Read the model definition and answer for the solid it produces. Units are mm, in the model's axes. Face numbers are marked on the shaded views. Give positions to 0.01 mm unless a question says otherwise; leave off trailing zeros. Write each loop counter-clockwise with the first axis right and the second up, starting at its lowest first coordinate (ties: lowest second). Pieces come first, ordered by that corner, then holes. Notation, with made-up numbers: (67, -35.5) - (110, -35.5) arc R21 ccw to (110, -12.5) - close; hole circle Ø2 at (-12, 46). An arc over 180 degrees is marked (long way). Answer as CSV lines item,"result".
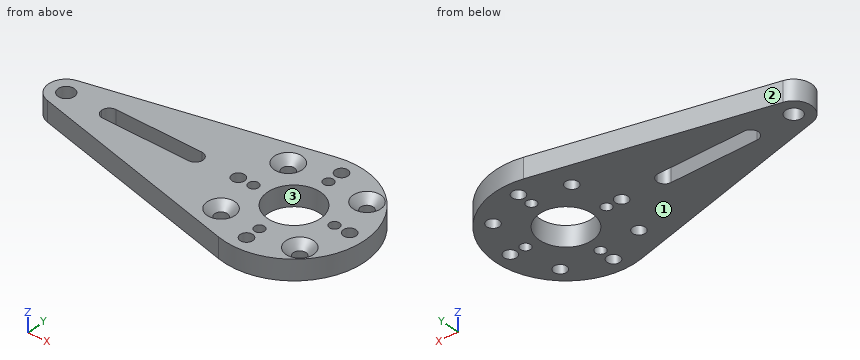
```python
from build123d import *

# Parameters (mm, degrees)
SKETCH1_R           = 1.6
SKETCH1_R_2         = 5.25
BOSS_EXTRUDE1_DEPTH = 4
CUT_EXTRUDE1_REACH  = 52.638
SKETCH2_R           = 1
CIRPATTERN1_COUNT   = 4
CUT_EXTRUDE2_REACH  = 52.638
SKETCH3_R           = 1.25
CIRPATTERN2_COUNT   = 8
CHAMFER1_SIZE       = 1.5
CUT_EXTRUDE3_REACH  = 52.638
SKETCH4_W           = 20
SKETCH4_H           = 3
FILLET1_R           = 1.5


with BuildPart() as part:
    # Sketch1 → Boss-Extrude1 (new body)
    with BuildSketch(Plane.XY):
        with BuildLine():
            Line((-45.816666667, 3.403388834), (-3.266666667, 13.613555336))
            ThreePointArc((-3.266666667, 13.613555336), (14, 0), (-3.266666667, -13.613555336))
            Line((-3.266666667, -13.613555336), (-45.816666667, -3.403388834))
            ThreePointArc((-45.816666667, -3.403388834), (-48.5, 0), (-45.816666667, 3.403388834))
        make_face()
        with Locations((-45, 0)):
            Circle(SKETCH1_R, mode=Mode.SUBTRACT)
        Circle(SKETCH1_R_2, mode=Mode.SUBTRACT)
    extrude(amount=BOSS_EXTRUDE1_DEPTH)

    # Sketch2 → Cut-Extrude1 (cut, up to next)
    with BuildSketch(Plane.XY.offset(4), mode=Mode.PRIVATE) as cut_extrude1_sk1:
        with Locations((0, 8)):
            Circle(SKETCH2_R)
    cut_extrude1_tool1 = extrude(cut_extrude1_sk1.sketch, amount=-CUT_EXTRUDE1_REACH, mode=Mode.PRIVATE) & part.part
    cut_extrude1 = cut_extrude1_tool1.solids().sort_by_distance((0, 8, 4))[0]
    add(cut_extrude1, mode=Mode.SUBTRACT)

    # CirPattern1: Cut-Extrude1 ×4 about axis
    cirpattern1_axis = Axis((0, 0, 0), (0, 0, 1))
    for i in range(1, CIRPATTERN1_COUNT):
        add(cut_extrude1.rotate(cirpattern1_axis, i * 360 / CIRPATTERN1_COUNT), mode=Mode.SUBTRACT)

    # Sketch3 → Cut-Extrude2 (cut, up to next)
    with BuildSketch(Plane.XY.offset(4), mode=Mode.PRIVATE) as cut_extrude2_sk1:
        with Locations((0, 11)):
            Circle(SKETCH3_R)
    cut_extrude2_tool1 = extrude(cut_extrude2_sk1.sketch, amount=-CUT_EXTRUDE2_REACH, mode=Mode.PRIVATE) & part.part
    cut_extrude2 = cut_extrude2_tool1.solids().sort_by_distance((0, 11, 4))[0]
    add(cut_extrude2, mode=Mode.SUBTRACT)

    # CirPattern2: Cut-Extrude2 ×8 about axis
    cirpattern2_axis = Axis((0, 0, 0), (0, 0, 1))
    for i in range(1, CIRPATTERN2_COUNT):
        add(cut_extrude2.rotate(cirpattern2_axis, i * 360 / CIRPATTERN2_COUNT), mode=Mode.SUBTRACT)

    # Chamfer1
    chamfer1_edges = [part.edges().sort_by_distance(p)[0] for p in [
        (-6.894291117, -8.66205807, 4),
        (8.66205807, -6.894291117, 4),
        (6.894291117, 8.66205807, 4),
        (-8.66205807, 6.894291117, 4),
    ]]
    chamfer(chamfer1_edges, length=CHAMFER1_SIZE)

    # Sketch4 → Cut-Extrude3 (cut, up to next)
    with BuildSketch(Plane.XY.offset(4), mode=Mode.PRIVATE) as cut_extrude3_sk1:
        with Locations((-28, 0)):
            Rectangle(SKETCH4_W, SKETCH4_H)
    cut_extrude3_tool1 = extrude(cut_extrude3_sk1.sketch, amount=-CUT_EXTRUDE3_REACH, mode=Mode.PRIVATE) & part.part
    add(cut_extrude3_tool1.solids().sort_by_distance((-28, 0, 4))[0], mode=Mode.SUBTRACT)

    # Fillet1
    fillet1_edges = [part.edges().sort_by_distance(p)[0] for p in [
        (-18, -1.5, 2),
        (-18, 1.5, 2),
        (-38, 1.5, 2),
        (-38, -1.5, 2),
    ]]
    fillet(fillet1_edges, radius=FILLET1_R - 0.0001)  # a hair under: the kernel refuses the full size


solid = part.part
```
(1) The mould has two halves that part along X. Classify the marked faces 1, 2 and 3: +X half, -X half, draft (parallel to the pull), parting line (faces both ways), or undercut.
Worked out:
face 1,"draft"
face 2,"-X half"
face 3,"undercut"
(2) Find the intervals of material crossed by L1, parallel to Y at x = 0, z = 0.85; L2, parallel to Y at x = -35, z = 0.85; L3, parallel to X at y = -1.75, z = 0.7, in increasing order.
Worked out:
L1,"y = -14 to -12.25, -9.75 to -9, -7 to -5.25, 5.25 to 7, 9 to 9.75, 12.25 to 14"
L2,"y = -6 to -1.5, 1.5 to 6"
L3,"x = -48.03 to -4.95, 4.95 to 13.89"
(3) A cutting plane is placed at A-A (x = -45). Write down the section's boundary in (y, z), and give its area (3 significant figures).
Worked out:
outline,"(-3.6, 0) - (-1.6, 0) - (-1.6, 4) - (-3.6, 4) - close; (1.6, 0) - (3.6, 0) - (3.6, 4) - (1.6, 4) - close"
area,"16.0 mm^2"
(4) A cutting plane is placed at B-B (z = 3.35). Count the separate pieces of the cut face and the enclosed holes in it, and give its area (3 significant figures).
Worked out:
separate pieces,"1"
enclosed holes,"15"
area,"896 mm^2"
(5) Each of these flat-tipped pins is pushed along its axis until it touches: P1, Ø1.2, axis at x = -29, z = 2.5, coming from the -Y side; P2, Ø1, axis at x = -14.5, z = 3.5, coming from the -Y side; P3, Ø1, axis at x = -41, z = 0.5, coming from the -Y side. Where does it stop, or does it pass through?
Worked out:
P1,"stops at y = -7.58"
P2,"stops at y = -11.04"
P3,"stops at y = -4.68"
(6) A cutting plane is placed at C-C (x = -28). Write down the section's boundary in (y, z).
Worked out:
outline,"(-7.68, 0) - (-1.5, 0) - (-1.5, 4) - (-7.68, 4) - close; (1.5, 0) - (7.68, 0) - (7.68, 4) - (1.5, 4) - close"
